Check sheet for the drawn part. Datum: minimum x, y, z corner. Units: mm. A direction names the side the tool comes from. Give positions to 0.01 mm unless a question says otherwise; leave off trailing zeros. Write each loop counter-clockwise with the first axis right and the second up, starting at its lowest first coordinate (ties: lowest second). Pieces come first, ordered by that corner, then holes. Notation, with made-up numbers: (60, 25) - (83, 25) arc R18 ccw to (83, 39) - close; hole circle Ø1 at (33, 11.5). An arc over 180 degrees is marked (long way). Use a Markdown table: item, result.
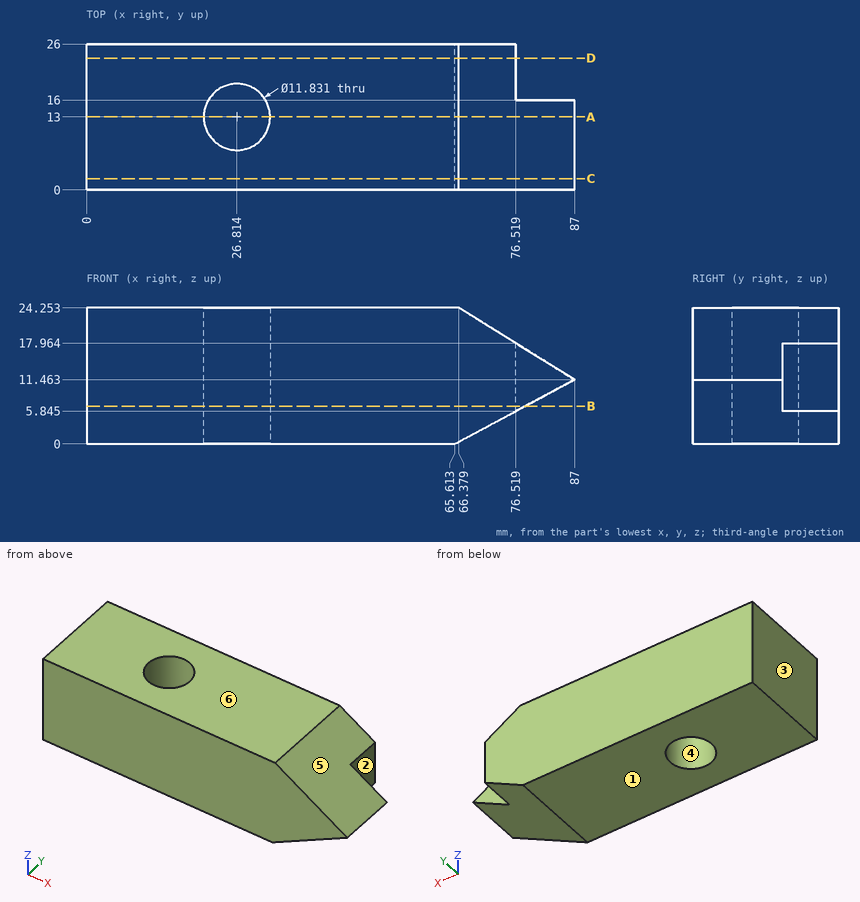
1) Section check B-B on z = 6.75. Record the boundary of the cut face in (x, y) (1 decimal), then the cut area to 3 significant figures.
Working result:
| item | result |
|---|---|
| outline | (0, 0) - (78.2, 0) - (78.2, 16) - (76.5, 16) - (76.5, 26) - (0, 26) - close; hole circle Ø11.8 at (26.8, 13) |
| area | 1,910 mm² |
2) Set-up check for the marked faces 1 and 2: record each of +Z, -Z, +X, -X, +Y, -Y from which the full face is reachable in a straight line by a thin tool's end or side.
Working result:
| item | result |
|---|---|
| face 1 | -Z, +X, -X, +Y, -Y |
| face 2 | +Z, -Z, +X, +Y |
3) Depth check by flat-ended pin: P1, Ø12, axis at x = 75, y = 3.5, coming from the -Z side (1 decimal); P2, Ø8, axis at x = 73.5, y = 11.5, coming from the +Z side; P3, Ø5, axis at x = 84, z = 12.5, coming from the +Y side. Enter the tip coordinate at first touch or a pass-through.
Working result:
| item | result |
|---|---|
| P1 | stops at z = 1.8 |
| P2 | stops at z = 22.32 |
| P3 | stops at y = 16 |
4) Section check A-A on y = 13. Record the boundary of the cut face in (x, z), then the cut area to 3 significant figures.
Working result:
| item | result |
|---|---|
| outline | (0, 0) - (20.9, 0) - (20.9, 24.25) - (0, 24.25) - close; (32.73, 0) - (65.61, 0) - (87, 11.46) - (66.38, 24.25) - (32.73, 24.25) - close |
| area | 1,570 mm² |
5) Material ranges on L1, parallel to X at y = 20.5, z = 23.25 (1 decimal); L2, parallel to Y at x = 31, z = 8.75; L3, parallel to X at y = 12, z = 7.75 (1 decimal), recorded low to high. Write a range as from..to.
Working result:
| item | result |
|---|---|
| L1 | x = 0..68 |
| L2 | y = 0..8.82, 17.18..26 |
| L3 | x = 0..21, 32.6..80.1 |
6) Mould release check, pull along X, two halves, no side actions. Record for the marked faces 3, 4, 5 and 6: pulls with the +X half, pulls with the -X half, needs draft (parallel to the pull), parting line crosses it, or undercut.
Working result:
| item | result |
|---|---|
| face 3 | pulls with the -X half |
| face 4 | undercut |
| face 5 | pulls with the +X half |
| face 6 | needs draft |
7) Section check D-D on y = 23.5. Record the boundary of the cut face in (x, z) (1 decimal), then the cut area to 3 significant figures.
Working result:
| item | result |
|---|---|
| outline | (0, 0) - (65.6, 0) - (76.5, 5.8) - (76.5, 18) - (66.4, 24.3) - (0, 24.3) - close |
| area | 1,790 mm² |
8) Section check C-C on y = 2. Record the boundary of the cut face in (x, z).
Working result:
| item | result |
|---|---|
| outline | (0, 0) - (65.61, 0) - (87, 11.46) - (66.38, 24.25) - (0, 24.25) - close |
